Work out the finished part from the listing and answer in its coordinate system (mm). Face numbers are marked on the shaded views. A direction names the side the tool comes from. Give positions to 0.01 mm unless a question says otherwise; leave off trailing zeros. Write each loop counter-clockwise with the first axis right and the second up, starting at its lowest first coordinate (ties: lowest second). Pieces come first, ordered by that corner, then holes.
1) Given pin 1 Ø9 at (x, z) = (33.77, -19.5) entering from -Y; pin 2 Ø13.5 at (x, z) = (0, -39) entering from -Y; pin 3 Ø12 at (x, z) = (11, -7.5) entering from +Y; pin 4 Ø1 at (x, y) = (-3.5, 3.5) entering from -Z, each flat-ended and moving along its own axis, determine where each tip first touches the part or whether it passes through.
2) Find section A-A (x = 0). Determine the outline of the cut face in (y, z).
3) A tool of negligible diameter and unlimited length cuts with its end or side. For the marked faces 1 and 2, from which of +Z, -Z, +X, -X, +Y, -Y can it reach the whole face along a straight path? Write none if from no direction.
4) Find section B-B (z = -9). Determine the outline of the cut face in (x, y).
5) Find section D-D (y = -3.75). Determine the outline of the cut face in (x, z).
6) Straight lines are drawn through the part: probe 1 along X at (y, z) = (2.55, 0); probe 2 along Y at (x, z) = (-9, 28.5); probe 3 along X at (y, z) = (-2.25, -10.5). For each, find the intervals that lie inside material, in ascending order.
7) Find section C-C (x = -34). Determine the outline of the cut face in (y, z), plus the area to 3 significant figures.
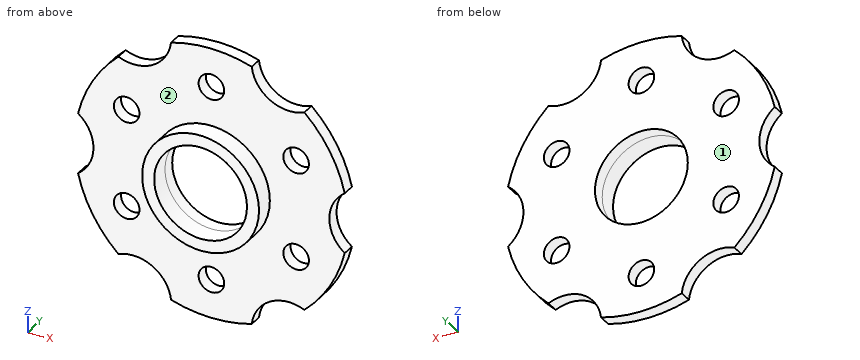
Autodesk Inventor part; units mm, degrees
ref_plane "YZ Plane" through (0, 0, 0) normal (1, 0, 0) x (0, 1, 0)
ref_plane "XZ Plane" through (0, 0, 0) normal (0, 1, 0) x (-1, 0, 0)
ref_plane "XY Plane" through (0, 0, 0) normal (0, 0, 1) x (1, 0, 0)
sketch "Sketch1" plane through (0, 0, 0) normal (0, 1, 0) x (-1, 0, 0)
  circle A0 centre (0, 0) radius 18.5
  circle A1 centre (0, 0) radius 39 construction
  circle A2 centre (0, -39) radius 5.1
  circle A3 centre (0, 0) radius 54.5
  circle A4 centre (0, 0) radius 62 construction
  circle A5 centre (-62, 0) radius 15
  dimension "d1" = 78
  dimension "d11" = 124
  dimension "d0" = 37
  dimension "d2" = 10.2
  dimension "d3" = 109
  dimension "d12" = 30
extrude "Extrusion1" add sketch "Sketch1" along normal blind 5 contours A2 | A3 A5 | A5 A3 picked at (16.1327, -31.6474) picked at (-51.8988, 0)
extrude "Extrusion2" cut sketch "Sketch1" along normal through all contours A2
pattern_circular "Circular Pattern1" count 6 over 360 about axis through (0, 0, 0) along (0, 1, 0) of "Extrusion2"
extrude "Extrusion3" cut sketch "Sketch1" along normal through all contours A5 A3 | A3 A5 picked at (-51.8988, 0) picked at (-61.8988, 0)
pattern_circular "Circular Pattern2" count 6 over 360 about axis through (0, 0, 0) along (0, 1, 0) of "Extrusion3"
sketch "Sketch2" plane through (0, 0, 0) normal (0, -1, 0) x (1, 0, 0)
  circle A0 centre (0, 0) radius 23.3
  circle A1 centre (0, 0) radius 18.5
  dimension "d18" = 46.6
  dimension "d19" = 37
extrude "Extrusion4" add sketch "Sketch2" along normal blind 7.5
properties part number "HELP_6204BEARING_CASE_B"
Results:
1. pin 1: passes through
1. pin 2: stops at y = 0
1. pin 3: stops at y = 5
1. pin 4: stops at z = -54.42
2. outline: (-7.5, -23.3) - (0, -23.3) - (0, -33.9) - (5, -33.9) - (5, -18.5) - (-7.5, -18.5) - close; (-7.5, 18.5) - (5, 18.5) - (5, 33.9) - (0, 33.9) - (0, 23.3) - (-7.5, 23.3) - close; (0, -54.5) - (5, -54.5) - (5, -44.1) - (0, -44.1) - close; (0, 44.1) - (5, 44.1) - (5, 54.5) - (0, 54.5) - close
3. face 1: +Z, -Z, +X, -X, +Y
3. face 2: -Y
4. outline: (-50, 0) - (-21.49, 0) - (-21.49, -7.5) - (-16.16, -7.5) - (-16.16, 5) - (-50, 5) - close; (16.16, -7.5) - (21.49, -7.5) - (21.49, 0) - (50, 0) - (50, 5) - (16.16, 5) - close
5. outline: circle Ø46.6 at (0, 0); hole circle Ø37 at (0, 0)
6. probe 1: x = -47 to -18.5, 18.5 to 47
6. probe 2: y = 0 to 5
6. probe 3: x = -20.8 to -15.23, 15.23 to 20.8
7. outline: (0, -39) - (5, -39) - (5, -24.6) - (0, -24.6) - close; (0, -14.4) - (5, -14.4) - (5, 14.4) - (0, 14.4) - close; (0, 24.6) - (5, 24.6) - (5, 39) - (0, 39) - close
7. area: 288 mm2
